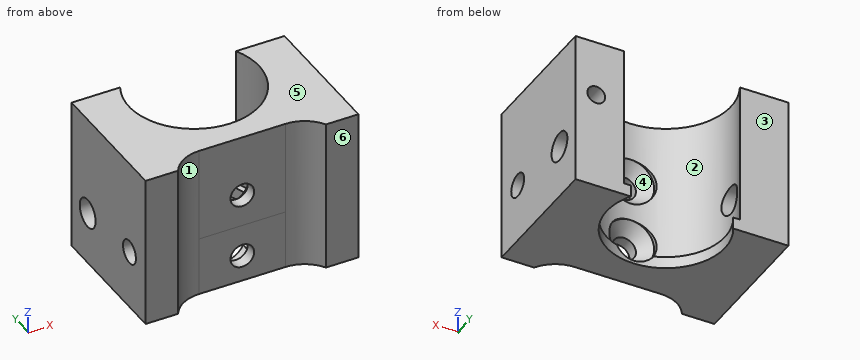
Autodesk Inventor part; units mm, degrees
ref_plane "Work Plane1" through (0, -5.5, 13) normal (0, 1, 0) x (-1, 0, 0)
ref_plane "YZ Plane" through (0, 0, 0) normal (1, 0, 0) x (0, 1, 0)
ref_plane "XZ Plane" through (0, 0, 0) normal (0, 1, 0) x (-1, 0, 0)
sketch "Sketch1" plane through (0, 0, 0) normal (0, 0, 1) x (1, 0, 0)
  arc A0 (-4.3301, 2.5) -> (4.3301, 2.5) centre (0, 0) ccw
  line L0 (-4.3301, 2.5) -> (-9, 2.5)
  line L1 (-9, 2.5) -> (-9, -9)
  line L2 (-9, -9) -> (-6.25, -9)
  line L3 (-3.6519, -7.5) -> (3.6519, -7.5)
  line L4 (6.25, -9) -> (9, -9)
  line L5 (9, -9) -> (9, 2.5)
  line L6 (9, 2.5) -> (4.3301, 2.5)
  line L7 (0, 15.116) -> (0, -11.4442) construction
  arc A1 (-3.6519, -7.5) -> (-6.25, -9) centre (-3.6519, -10.5) ccw
  arc A2 (6.25, -9) -> (3.6519, -7.5) centre (3.6519, -10.5) ccw
  dimension "d0" = 10
  dimension "d2" = 7.5
  dimension "d5" = 18
  dimension "d6" = 2.5
  dimension "d7" = 6
  dimension "d8" = 6
  dimension "d9" = 12.5
  dimension "d10" = 1.5
sketch "Sketch2" plane through (0, 0, 0) normal (0, 0, 1) x (1, 0, 0)
  line L0 (-4.3301, 2.5) -> (-9, 2.5)
  line L1 (-9, 2.5) -> (-9, -9)
  line L2 (-9, -9) -> (-6.25, -9)
  arc A0 (-3.6519, -7.5) -> (-6.25, -9) centre (-3.6519, -10.5) ccw
  line L3 (-3.6519, -7.5) -> (3.6519, -7.5)
  arc A1 (6.25, -9) -> (3.6519, -7.5) centre (3.6519, -10.5) ccw
  line L4 (6.25, -9) -> (9, -9)
  line L5 (9, -9) -> (9, 2.5)
  line L6 (9, 2.5) -> (4.3301, 2.5)
  arc A2 (-4.3301, 2.5) -> (4.3301, 2.5) centre (0, 0) ccw
extrude "Extrusion1" add sketch "Sketch2" along normal blind 13
sketch "Sketch3" plane through (0, 0, 13) normal (0, 0, 1) x (1, 0, 0)
  circle A0 centre (0, 0) radius 5.5
  dimension "d13" = 11
extrude "Extrusion2" cut sketch "Sketch3" against normal blind 12
sketch "Sketch4" plane through (-9, 2.5, 0) normal (0, 1, 0) x (1, 0, 0)
  line L0 (9, 0) -> (9, -15.5) construction
  line L1 (18, -13) -> (13.899, -13)
  line L2 (14.5, -13) -> (3.5, -13)
  point P0 (9, -2.25)
  point P1 (9, -7.75)
  point P2 (16.25, -8.25)
  point P3 (4.101, -13)
  dimension "d16" = 7.25
  dimension "d17" = 4.75
  dimension "d18" = 5.25
  dimension "d19" = 5.5
sketch "Sketch5" plane through (4.3301, 2.5, 0) normal (0, 1, 0) x (1, 0, 0)
  point P0 (-4.3301, 0)
  point P1 (2.9199, -8.25)
hole "Hole1" at (7.25, 2.5, 8.25) direction (0, -1, 0) diameter 1.5 depth 5 tip angle 118
ref_plane "Work Plane1" through (0, -5.5, 13) normal (0, 1, 0) x (-1, 0, 0)
sketch "Sketch6" plane through (-9, 2.5, 0) normal (0, 1, 0) x (1, 0, 0)
  point P0 (9, 0)
  point P1 (9, -2.25)
  point P2 (9, -7.75)
hole "Hole2" at (0, 2.5, 7.75) at (0, 2.5, 2.25) direction (0, -1, 0) diameter 4 depth 8
sketch "Sketch7" plane through (0, -5.5, 13) normal (0, 1, 0) x (-1, 0, 0)
  point P0 (0, -13)
  point P1 (0, -10.75)
  point P2 (0, -5.25)
hole "Hole3" at (0, -5.5, 2.25) at (0, -5.5, 7.75) direction (0, -1, 0) diameter 2 end through all countersink diameter 4 countersink angle 90
sketch "Sketch8" plane through (-9, -9, 0) normal (-1, 0, 0) x (0, 0, 1)
  line L0 (0, 11.5) -> (13, 11.5)
  line L1 (0, 11.5) -> (0, 0)
  point P0 (0, 9)
  point P1 (5, 2.5)
  point P2 (4.5, 9)
  dimension "d41" = 9
  dimension "d42" = 5
  dimension "d43" = 2.5
  dimension "d44" = 4.5
sketch "Sketch9" plane through (-9, -9, 0) normal (-1, 0, 0) x (0, 0, 1)
  point P0 (0, 9)
  point P1 (5, 2.5)
hole "Hole4" at (-9, -6.5, 5) direction (1, 0, 0) diameter 2 end through all
sketch "Sketch10" plane through (-9, -9, 0) normal (-1, 0, 0) x (0, 0, 1)
  point P0 (0, 9)
  point P1 (4.5, 9)
hole "Hole5" at (-9, 0, 4.5) direction (1, 0, 0) diameter 2.459 end through all
equation "\"d7\" = d8"
properties part number "trolley"
Check sheet for the modelled part. Datum: model origin and axes. Units: mm. Face numbers are marked on the shaded views. A direction names the side the tool comes from. Round coordinates to 2 decimals unless told otherwise and drop trailing zeros. Loops run counter-clockwise (first coordinate to the right, second up) from the corner with the lowest first, then second, coordinate; pieces in that order, holes last. Notation, with made-up numbers: (-29, 79) -> (22, 79) arc R22 ccw to (22, 95) -> close; hole circle Ø5 at (85, 45.5). An arc over 180 degrees is marked (long way). Put each result on its own line as item: value. Start each with the question number.
1. Section check B-B (z = 2.25). Enter the section's corners in (x, y), plus the area to 3 significant figures.
2. Section check C-C (y = 1.5). Enter the section's corners in (x, z), plus the area to 3 significant figures.
3. Section check A-A (y = 0). Enter the section's corners in (x, z).
4. Draft check along Z on the marked faces 4, 5 and 6. Enter one of: +Z half, -Z half, draft (parallel to the pull), parting line (faces both ways), or undercut.
5. Scan lines: probe 1 along X at (y, z) = (-5.15, 2.25); probe 2 along Y at (x, z) = (0, 10); probe 3 along X at (y, z) = (-3.25, 11). Record each from-to range of solid material in increasing order.
6. Section check D-D (x = -7.5). Enter the section's corners in (y, z).
7. Gauge pin test, flat ends, axial feed: pin 1 (3 mm diameter, centred on x = 0, z = 2.25, fed in from -Y); pin 2 (1.4 mm diameter, centred on x = 7.25, z = 8.25, fed in from +Y); pin 3 (2.5 mm diameter, centred on x = 0, z = 7.75, fed in from +Y). Record the tip position at first contact, or that the pin passes through.
8. Access from +Z, -Z, +X, -X, +Y, -Y to the whole of each face (thin tool, end or side, straight path). Record for the marked faces 1, 2 and 3.
Findings:
1. outline: (-9, -9) -> (-6.25, -9) arc R3 cw to (-3.65, -7.5) -> (-1, -7.5) -> (-1, -6.5) -> (-2, -5.5) -> (-2, -5.12) arc R5.5 cw to (-4.9, 2.5) -> (-9, 2.5) -> close; (1, -7.5) -> (3.65, -7.5) arc R3 cw to (6.25, -9) -> (9, -9) -> (9, 2.5) -> (4.9, 2.5) arc R5.5 cw to (2, -5.12) -> (2, -5.5) -> (1, -6.5) -> close
1. area: 111 mm^2
2. outline: (-9, 0) -> (-4.77, 0) -> (-4.77, 1) -> (-5.29, 1) -> (-5.29, 13) -> (-9, 13) -> close; (4.77, 0) -> (9, 0) -> (9, 13) -> (5.29, 13) -> (5.29, 1) -> (4.77, 1) -> close; hole circle Ø1.5 at (7.25, 8.25)
2. area: 95.7 mm^2
3. outline: (-9, 0) -> (-5, 0) -> (-5, 1) -> (-5.5, 1) -> (-5.5, 3.27) -> (-9, 3.27) -> close; (-9, 5.73) -> (-5.5, 5.73) -> (-5.5, 13) -> (-9, 13) -> close; (5, 0) -> (9, 0) -> (9, 3.27) -> (5.5, 3.27) -> (5.5, 1) -> (5, 1) -> close; (5.5, 5.73) -> (9, 5.73) -> (9, 13) -> (5.5, 13) -> close; hole circle Ø1.5 at (7.25, 8.25)
4. face 4: undercut
4. face 5: +Z half
4. face 6: draft
5. probe 1: x = -9 to -2, 2 to 9
5. probe 2: y = -7.5 to -5.5
5. probe 3: x = -9 to -4.44, 4.44 to 9
6. outline: (-9, 0) -> (2.5, 0) -> (2.5, 13) -> (-9, 13) -> close; hole circle Ø2 at (-6.5, 5); hole circle Ø2.46 at (0, 4.5)
7. pin 1: stops at y = -7.5
7. pin 2: stops at y = -2.53
7. pin 3: stops at y = -6.25
8. face 1: +Z, -Z, -Y
8. face 2: +Z
8. face 3: +Z, -Z, +X, -X, +Y
